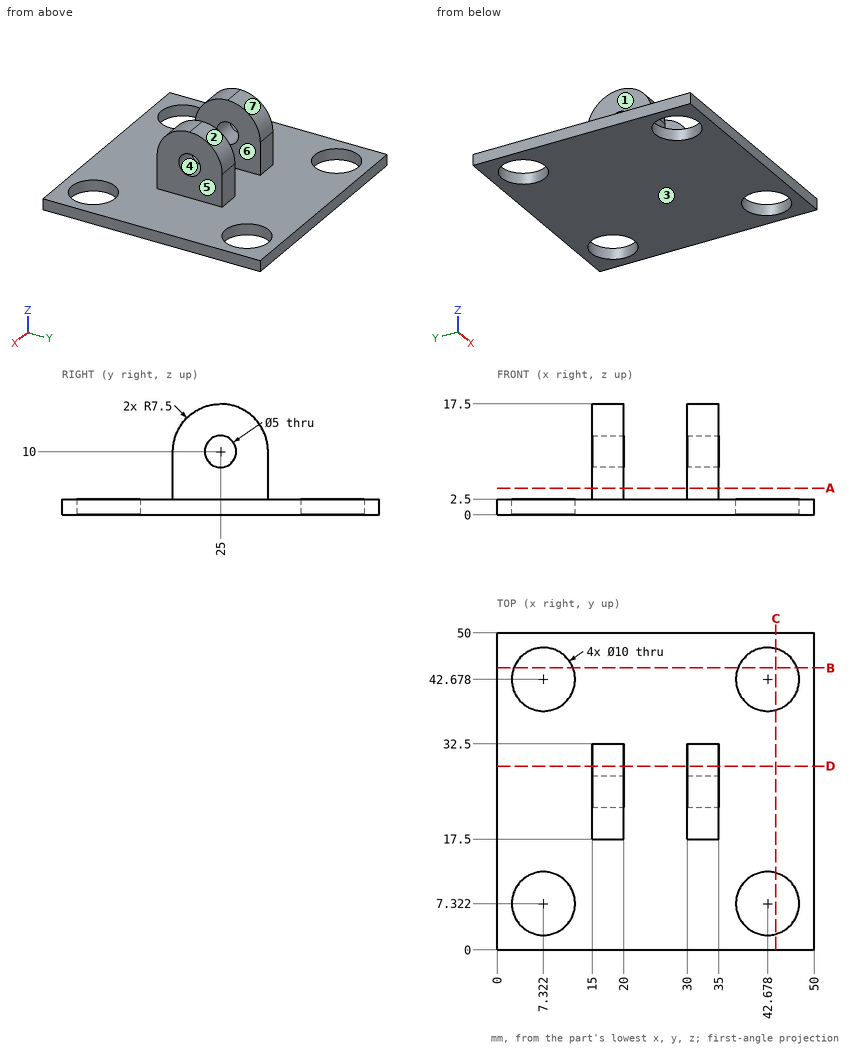
Geometry check sheet. Reference: drawing and pictorial views, mm from the part's lowest x, y, z. A direction names the side the tool comes from. Coordinates: 2 decimals unless noted, no trailing zeros. Order: outer loops, then holes, each group sorted by start corner. A loop starts at its lowest first (then second) coordinate and runs counter-clockwise, first axis right, second up.
Item 1: Section check A-A, the plane z = 4.25. Enter the section's corners in (x, y).
Filled in:
outline: (15, 17.5) - (20, 17.5) - (20, 32.5) - (15, 32.5) - close; (30, 17.5) - (35, 17.5) - (35, 32.5) - (30, 32.5) - close
Item 2: Section check C-C, the plane x = 44. Enter the section's corners in (y, z).
Filled in:
outline: (0, 0) - (2.5, 0) - (2.5, 2.5) - (0, 2.5) - close; (12.14, 0) - (37.86, 0) - (37.86, 2.5) - (12.14, 2.5) - close; (47.5, 0) - (50, 0) - (50, 2.5) - (47.5, 2.5) - close
Item 3: Depth check by flat-ended pin: pin 1 (25 mm diameter, centred on x = 28, y = 36, fed in from +Z); pin 2 (2.5 mm diameter, centred on x = 18.5, z = 8, fed in from -Y); pin 3 (3 mm diameter, centred on x = 30, z = 13.5, fed in from -Y); pin 4 (12 mm diameter, centred on x = 41, y = 36.5, fed in from +Z). Enter the tip coordinate at first touch or a pass-through.
Filled in:
pin 1: stops at z = 17.5
pin 2: stops at y = 17.5
pin 3: stops at y = 17.77
pin 4: stops at z = 2.5
Item 4: Section check B-B, the plane y = 44.5. Enter the section's corners in (x, z).
Filled in:
outline: (0, 0) - (2.67, 0) - (2.67, 2.5) - (0, 2.5) - close; (11.98, 0) - (38.02, 0) - (38.02, 2.5) - (11.98, 2.5) - close; (47.33, 0) - (50, 0) - (50, 2.5) - (47.33, 2.5) - close
Item 5: Section check D-D, the plane y = 29. Enter the section's corners in (x, z) (1 decimal).
Filled in:
outline: (0, 0) - (50, 0) - (50, 2.5) - (35, 2.5) - (35, 16.3) - (30, 16.3) - (30, 2.5) - (20, 2.5) - (20, 16.3) - (15, 16.3) - (15, 2.5) - (0, 2.5) - close
Item 6: Material ranges on L1, parallel to X at y = 8, z = 1.5; L2, parallel to Z at x = 36, y = 26; L3, parallel to X at y = 21.5, z = 12, recorded low to high.
Filled in:
L1: x = 0 to 2.37, 12.28 to 37.72, 47.63 to 50
L2: z = 0 to 2.5
L3: x = 15 to 20, 30 to 35
Item 7: Access from +Z, -Z, +X, -X, +Y, -Y to the whole of each face (thin tool, end or side, straight path). Record for the marked faces 5, 6 and 7.
Filled in:
face 5: +Z, +X, +Y, -Y
face 6: +Z, +Y, -Y
face 7: +Z, +X, -X, +Y
Item 8: Release check for a two-part mould opening along Z. For the marked faces 1, 2, 3 and 4 record: +Z half, -Z half, draft (parallel to the pull), parting line (faces both ways), or undercut.
Filled in:
face 1: draft
face 2: +Z half
face 3: -Z half
face 4: undercut
